```python
from build123d import *

# Parameters (mm, degrees)
SKETCH1_R               = 21.5
BOSS_EXTRUDE1_DEPTH     = 3
BOSS_EXTRUDE2_START     = 3
SKETCH1_3_R             = 21.5
SKETCH1_3_R_2           = 18.5
BOSS_EXTRUDE2_DEPTH     = 20
CUT_EXTRUDE1_DEPTH      = 39.124795081
CUT_EXTRUDE1_DEPTH_BACK = 39.124795081
SKETCH3_R               = 6.25
SKETCH3_R_2             = 1.3
BOSS_EXTRUDE3_START     = 19
SKETCH4_R               = 1.35
BOSS_EXTRUDE3_DEPTH     = 4
FILLET1_R               = 1


with BuildPart() as part:
    # Sketch1 → Boss-Extrude1 (new body)
    with BuildSketch(Plane.XY):
        Circle(SKETCH1_R)
    extrude(amount=BOSS_EXTRUDE1_DEPTH)

    # Sketch1<3> → Boss-Extrude2 (add)
    with BuildSketch(Plane.XY.offset(BOSS_EXTRUDE2_START)):
        Circle(SKETCH1_3_R)
        Circle(SKETCH1_3_R_2, mode=Mode.SUBTRACT)
    extrude(amount=BOSS_EXTRUDE2_DEPTH)

    # Sketch3 → Cut-Extrude1 (cut, two sides: drawn at the far end of the back side and taken through both)
    with BuildSketch(Plane.XY.offset(-CUT_EXTRUDE1_DEPTH_BACK)):
        with Locations((0, -7)):
            Circle(SKETCH3_R)
        with Locations((7.75, 13.423393759)):
            Circle(SKETCH3_R_2)
        with Locations((-7.75, 13.423393759)):
            Circle(SKETCH3_R_2)
        with Locations((15.5, 0)):
            Circle(SKETCH3_R_2)
        with Locations((-15.5, 0)):
            Circle(SKETCH3_R_2)
        with Locations((7.75, -13.423393759)):
            Circle(SKETCH3_R_2)
        with Locations((-7.75, -13.423393759)):
            Circle(SKETCH3_R_2)
    extrude(amount=CUT_EXTRUDE1_DEPTH + CUT_EXTRUDE1_DEPTH_BACK, mode=Mode.SUBTRACT)

    # Sketch4 → Boss-Extrude3 (add)
    # profile 1 of 4: a face of its own
    with BuildSketch(Plane.XY.offset(BOSS_EXTRUDE3_START)):
        with BuildLine():
            Line((-17.175389561, 12.932748874), (-20.710923467, 16.46828278))
            ThreePointArc((-20.710923467, 16.46828278), (-21.589603123, 18.589603123), (-20.710923467, 20.710923467))
            ThreePointArc((-20.710923467, 20.710923467), (-18.589603123, 21.589603123), (-16.46828278, 20.710923467))
            Line((-16.46828278, 20.710923467), (-12.932748874, 17.175389561))
            ThreePointArc((-12.932748874, 17.175389561), (-15.202795796, 15.202795796), (-17.175389561, 12.932748874))
        make_face()
        with Locations((-18.589603123, 18.589603123)):
            Circle(SKETCH4_R, mode=Mode.SUBTRACT)
    # profile 2 of 4: a face of its own
    with BuildSketch(Plane.XY.offset(BOSS_EXTRUDE3_START)):
        with BuildLine():
            Line((12.932748874, 17.175389561), (16.46828278, 20.710923467))
            ThreePointArc((16.46828278, 20.710923467), (18.589603123, 21.589603123), (20.710923467, 20.710923467))
            ThreePointArc((20.710923467, 20.710923467), (21.589603123, 18.589603123), (20.710923467, 16.46828278))
            Line((20.710923467, 16.46828278), (17.175389561, 12.932748874))
            ThreePointArc((17.175389561, 12.932748874), (15.202795796, 15.202795796), (12.932748874, 17.175389561))
        make_face()
        with Locations((18.589603123, 18.589603123)):
            Circle(SKETCH4_R, mode=Mode.SUBTRACT)
    # profile 3 of 4: a face of its own
    with BuildSketch(Plane.XY.offset(BOSS_EXTRUDE3_START)):
        with BuildLine():
            Line((17.175389561, -12.932748874), (20.710923467, -16.46828278))
            ThreePointArc((20.710923467, -16.46828278), (21.589603123, -18.589603123), (20.710923467, -20.710923467))
            ThreePointArc((20.710923467, -20.710923467), (18.589603123, -21.589603123), (16.46828278, -20.710923467))
            Line((16.46828278, -20.710923467), (12.932748874, -17.175389561))
            ThreePointArc((12.932748874, -17.175389561), (15.202795796, -15.202795796), (17.175389561, -12.932748874))
        make_face()
        with Locations((18.589603123, -18.589603123)):
            Circle(SKETCH4_R, mode=Mode.SUBTRACT)
    # profile 4 of 4: a face of its own
    with BuildSketch(Plane.XY.offset(BOSS_EXTRUDE3_START)):
        with BuildLine():
            Line((-12.932748874, -17.175389561), (-16.46828278, -20.710923467))
            ThreePointArc((-16.46828278, -20.710923467), (-18.589603123, -21.589603123), (-20.710923467, -20.710923467))
            ThreePointArc((-20.710923467, -20.710923467), (-21.589603123, -18.589603123), (-20.710923467, -16.46828278))
            Line((-20.710923467, -16.46828278), (-17.175389561, -12.932748874))
            ThreePointArc((-17.175389561, -12.932748874), (-15.202795796, -15.202795796), (-12.932748874, -17.175389561))
        make_face()
        with Locations((-18.589603123, -18.589603123)):
            Circle(SKETCH4_R, mode=Mode.SUBTRACT)
    extrude(amount=BOSS_EXTRUDE3_DEPTH)

    # Fillet1
    fillet1_edges = [part.edges().sort_by_distance(p)[0] for p in [
        (-17.175389561, -12.932748874, 21),
        (-12.932748874, -17.175389561, 21),
        (-15.202795796, -15.202795796, 19),
        (-12.932748874, 17.175389561, 21),
        (-17.175389561, 12.932748874, 21),
        (-15.202795796, 15.202795796, 19),
        (17.175389561, 12.932748874, 21),
        (12.932748874, 17.175389561, 21),
        (15.202795796, 15.202795796, 19),
        (12.932748874, -17.175389561, 21),
        (17.175389561, -12.932748874, 21),
        (15.202795796, -15.202795796, 19),
    ]]
    fillet(fillet1_edges, radius=FILLET1_R)


solid = part.part
```
Model file for the job. Use its own axes, mm. A direction names the side the tool comes from. Coordinates: 2 decimals unless noted, no trailing zeros. Loops run counter-clockwise (first coordinate to the right, second up) from the corner with the lowest first, then second, coordinate; pieces in that order, holes last. Notation, with made-up numbers: M 40,73.25 L 62,73.25 A34 ccw 62,112.25 Z; hole C -3.75,79.25 d9. An arc over 180 degrees is marked long. Use CSV: the item, a comma, the result in double quotes. Start each with the question number.
1. Two-plate mould, pull along Y, no slides. Class faces 4 (the flat face through (19.22, -14.98, 20.97)), 5 (the flat face through (18, -17, 19)), 6 (the cylindrical face through (12.91, 17.49, 20.54)): pulls with the +Y half, pulls with the -Y half, needs draft (parallel to the pull), parting line crosses it, or undercut.
2. Flat gauge pins, fed straight in: pin 1 (4 mm diameter, centred on x = -18, y = -15.5, fed in from -Z); pin 2 (1 mm diameter, centred on y = 0.5, z = 8, fed in from -X); pin 3 (6 mm diameter, centred on y = 8, z = 12, fed in from -X). Where does each tip first touch, or does it go through?
3. Tool access for faces 1 (the flat face through (19.26, 15.02, 20.97)), 2 (the flat face through (-18, 17, 19)), 3 (the flat face through (15.02, -19.26, 20.97)): list every direction of +Z, -Z, +X, -X, +Y, -Y with a clear straight run to the whole face (end or side of a thin tool).
4. Band-saw the part on B-B, the plane y = 0. List the corners of the cut face in (x, z).
5. Probe probe 1 along Z at (x, y) = (6, -0.5); probe 2 along Y at (x, z) = (11.5, 9.5); probe 3 along X at (y, z) = (-12.5, 21.25). List the from-to ranges inside material, lowest first. Write a range as [from, to].
6. Band-saw the part on C-C, the plane x = -7.75. List the corners of the cut face in (y, z).
7. Band-saw the part on D-D, the plane z = 13.25. List the corners of the cut face in (x, y).
8. Band-saw the part on A-A, the plane x = 0. List the corners of the cut face in (y, z), then the cut area to 4 significant figures.
Entries:
1,face 4,"undercut"
1,face 5,"needs draft"
1,face 6,"pulls with the +Y half"
2,pin 1,"stops at z = 18.67"
2,pin 2,"stops at x = -21.5"
2,pin 3,"stops at x = -20.91"
3,face 1,"+Z, -Z, +X"
3,face 2,"-Z, -X, +Y"
3,face 3,"+Z, -Z, -Y"
4,outline,"M -21.5,0 L -16.8,0 L -16.8,3 L -18.5,3 L -18.5,23 L -21.5,23 Z; M -14.2,0 L 14.2,0 L 14.2,3 L -14.2,3 Z; M 16.8,0 L 21.5,0 L 21.5,23 L 18.5,23 L 18.5,3 L 16.8,3 Z"
5,probe 1,"z = [0, 3]"
5,probe 2,"y = [-18.17, -14.49], [14.49, 18.17]"
5,probe 3,"x = [-17.54, -13.64], [13.64, 17.54]"
6,outline,"M -20.05,0 L -14.72,0 L -14.72,3 L -16.8,3 L -16.8,23 L -20.05,23 Z; M -12.12,0 L 12.12,0 L 12.12,3 L -12.12,3 Z; M 14.72,0 L 20.05,0 L 20.05,23 L 16.8,23 L 16.8,3 L 14.72,3 Z"
7,outline,"C 0,0 d43; hole C 0,0 d37"
8,outline,"M -21.5,0 L -13.25,0 L -13.25,3 L -18.5,3 L -18.5,23 L -21.5,23 Z; M -0.75,0 L 21.5,0 L 21.5,23 L 18.5,23 L 18.5,3 L -0.75,3 Z"
8,area,"211.5 mm2"
